Could you check a few things on this model? Use its own coordinates, in mm. Face numbers are marked on the shaded views. A direction names the side the tool comes from. Give positions to 0.01 mm unless a question says otherwise; leave off trailing zeros. Order: outer loops, then holes, each group sorted by start corner. A loop starts at its lowest first (then second) coordinate and runs counter-clockwise, first axis right, second up. Notation, with made-up numbers: (-16.5, 20.25) - (-8.5, 20.25) arc R13 cw to (-8.5, 30.25) - close; hole circle Ø8 at (45, 82.5). An arc over 180 degrees is marked (long way). Put each result on its own line as item: value.
Autodesk Inventor part; units mm, degrees
ref_plane "Work Plane2" through (10, 17.3205, 5.1062) normal (0.5, 0.866, 0) x (-0.866, 0.5, 0)
ref_plane "XZ Plane" through (0, 0, 0) normal (0, 1, 0) x (-1, 0, 0)
ref_plane "XY Plane" through (0, 0, 0) normal (0, 0, 1) x (1, 0, 0)
sketch "Sketch1" plane through (0, 0, 0) normal (1, 0, 0) x (0, 1, 0)
  line L0 (0, 0) -> (0, -33.1818)
  line L1 (4.5, 10.1062) -> (20, 10.1062)
  line L2 (20, 10.1062) -> (20, 0.1062)
  line L3 (20, 0.1062) -> (7.5, 0.1062)
  line L4 (7.5, 0.1062) -> (7.5, -29.8938)
  line L5 (7.5, -29.8938) -> (4.5, -29.8938)
  line L6 (4.5, -29.8938) -> (4.5, 10.1062)
  line L7 (7.5, 10.1062) -> (7.5, 40.1062)
  line L8 (7.5, 40.1062) -> (4.5, 40.1062)
  line L9 (4.5, 40.1062) -> (4.5, 10.1062)
  dimension "d0" = 9
  dimension "d1" = 15
  dimension "d2" = 30
  dimension "d3" = 10
  dimension "d4" = 40
  dimension "d28" = 30
revolve "Revolution1" add sketch "Sketch1" angle 360 about axis through (0, 0, 0) along (0, 0, -1)
sketch "Sketch2" plane through (0, 0, 10.1062) normal (0, 0, 1) x (1, 0, 0)
  point P0 (0, 0)
  point P1 (0, 16)
  dimension "d6" = 16
hole "Hole1" at (0, 16, 10.1062) direction (0, 0, -1) diameter 5 end through all
pattern_circular "Circular Pattern1" count 6 over 360 about axis through (0, 0, 5.1062) along (0, 0, -1) of "Hole1"
ref_plane "Work Plane2" through (10, 17.3205, 5.1062) normal (0.5, 0.866, 0) x (-0.866, 0.5, 0)
ref_plane "Work Plane1" through (0, 0, 0) normal (0.5, 0.866, 0) x (0, 0, 1)
sketch "Sketch3" plane through (10, 17.3205, 5.1062) normal (0.5, 0.866, 0) x (-0.866, 0.5, 0)
  line L0 (-20, 5) -> (20, 5)
  line L1 (-20, -5) -> (20, -5)
  line L2 (0, 5) -> (0, -5.1062)
  point P0 (0, -0.0531)
hole "Hole2" at (10, 17.3205, 5.0531) direction (-0.5, -0.866, 0) diameter 6.647 depth 20.2 tip angle 118
chamfer "Chamfer1" distance 0.2 angle 45 5 edges at (0, -20, 0.1062) (0, -20, 10.1062) (0, -7.5, -29.8938) (0, -7.5, 40.1062) (0, -4.5, 40.1062)
equation "\"d28\" = d2"
properties part number "Anode" material "Copper"
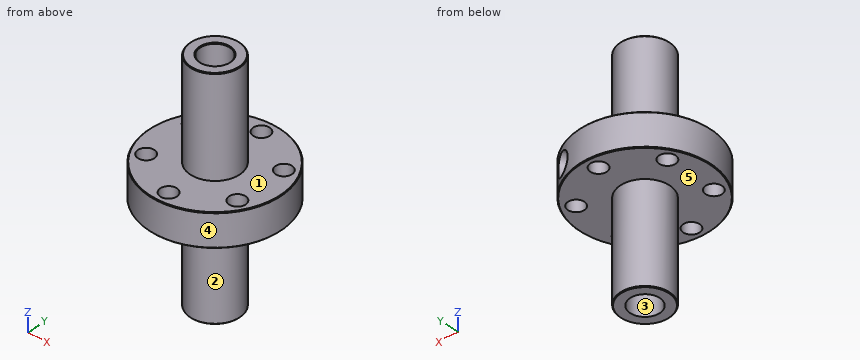
1) Which directions (+Z, -Z, +X, -X, +Y, -Y) give clear straight access to the entire face, cutting with the end or side of a thin tool? Please do the marked faces 1 and 2.
Filled in:
face 1: +Z
face 2: -Z
2) Suppose I cut it at C-C, the plane z = -1.5. List the corners of the cut face in (x, y) for me.
Filled in:
outline: circle Ø15 at (0, 0); hole circle Ø9 at (0, 0)
3) We'd pull the mould along X, two halves only. Please class the marked faces 3, 4 and 5: pulls with the +X half, pulls with the -X half, needs draft (parallel to the pull), parting line crosses it, or undercut.
Filled in:
face 3: undercut
face 4: parting line crosses it
face 5: needs draft
4) Suppose I cut it at B-B, the plane z = 6. List the corners of the cut face in (x, y) for me, and give its area (3 significant figures).
Filled in:
outline: (-1.17, 4.35) - (7.11, 18.69) arc R20 ccw (long way) to (12.63, 15.51) - (4.35, 1.16) arc R4.5 cw (long way) to start; hole circle Ø5 at (-13.86, -8); hole circle Ø5 at (-13.86, 8); hole circle Ø5 at (0, -16); hole circle Ø5 at (0, 16); hole circle Ø5 at (13.86, -8); hole circle Ø5 at (13.86, 8)
area: 974 mm^2
5) Suppose I cut it at D-D, the plane x = 0. State how many separate pieces and enclosed holes the cut face has, and give its area (3 significant figures).
Filled in:
separate pieces: 4
enclosed holes: 0
area: 563 mm^2
6) Suppose I cut it at A-A, the plane y = 0. List the corners of the cut face in (x, z) for me, and give its area (3 significant figures).
Filled in:
outline: (-20, 0.31) - (-19.8, 0.11) - (-7.5, 0.11) - (-7.5, -29.69) - (-7.3, -29.89) - (-4.5, -29.89) - (-4.5, 39.91) - (-4.7, 40.11) - (-7.3, 40.11) - (-7.5, 39.91) - (-7.5, 10.11) - (-19.8, 10.11) - (-20, 9.91) - close; (4.5, -29.89) - (7.3, -29.89) - (7.5, -29.69) - (7.5, 0.11) - (19.8, 0.11) - (20, 0.31) - (20, 9.91) - (19.8, 10.11) - (7.5, 10.11) - (7.5, 39.91) - (7.3, 40.11) - (4.7, 40.11) - (4.5, 39.91) - close
area: 670 mm^2
7) If I drill on line 1 (X direction, y = -8, z = 3.75); line 2 (Z direction, x = -6, y = -5.5); line 3 (X direction, y = 8, z = 3), over which ranges is the centre line in solid material (lowest first)? Write a range as [from, to].
Filled in:
line 1: x = [-18.33, -16.36], [-11.36, 11.36], [16.36, 18.33]
line 2: z = [0.11, 10.11]
line 3: x = [-18.33, -16.36], [-11.36, 1.6], [7.64, 11.36], [16.36, 18.33]
8) I'm going to push flat-ended pins straight in: pin 1 (4 mm diameter, centred on x = 0, y = 16, fed in from -Z); pin 2 (2 mm diameter, centred on x = -7.5, y = -7, fed in from -Z); pin 3 (6 mm diameter, centred on x = 4, y = 2, fed in from -Z); pin 4 (3 mm diameter, centred on x = -3.5, y = 8.5, fed in from +Z). Where does each tip first touch, or does it pass through?
Filled in:
pin 1: passes through
pin 2: stops at z = 0.11
pin 3: stops at z = -29.89
pin 4: stops at z = 10.11
